from build123d import *

# Parameters (mm, degrees)
SKETCH1_W           = 153
SKETCH1_H           = 72
SKETCH1_R           = 2.5
BOSS_EXTRUDE1_DEPTH = 8
SKETCH2_R           = 4.5
SKETCH2_R_2         = 2.1
BOSS_EXTRUDE2_DEPTH = 5
CHAMFER1_SIZE       = 5
SKETCH3_R           = 2.1
CUT_EXTRUDE1_DEPTH  = 5


with BuildPart() as part:
    # Sketch1 → Boss-Extrude1 (new body)
    with BuildSketch(Plane.XY):
        with Locations((76.5, 36)):
            Rectangle(SKETCH1_W, SKETCH1_H)
        with Locations((21.5, 61)):
            Circle(SKETCH1_R, mode=Mode.SUBTRACT)
        with Locations(Location((21.5, 11, 0), (0, 0, 180))):
            Circle(SKETCH1_R, mode=Mode.SUBTRACT)
        with Locations(Location((131.5, 61, 0), (0, 0, 180))):
            Circle(SKETCH1_R, mode=Mode.SUBTRACT)
        with Locations((131.5, 11)):
            Circle(SKETCH1_R, mode=Mode.SUBTRACT)
        with Locations((61.5, 61)):
            Circle(SKETCH1_R, mode=Mode.SUBTRACT)
        with Locations((46.5, 61)):
            Circle(SKETCH1_R, mode=Mode.SUBTRACT)
        with Locations(Location((106.5, 61, 0), (0, 0, 180))):
            Circle(SKETCH1_R, mode=Mode.SUBTRACT)
        with Locations(Location((91.5, 61, 0), (0, 0, 180))):
            Circle(SKETCH1_R, mode=Mode.SUBTRACT)
    extrude(amount=BOSS_EXTRUDE1_DEPTH)

    # Sketch2 → Boss-Extrude2 (add)
    # profile 1 of 4: a face of its own
    with BuildSketch(Plane.XY.offset(8)):
        with Locations(Location((12.5, 59.5, 0), (0, 0, 180))):
            Circle(SKETCH2_R)
        with Locations((12.5, 59.5)):
            Circle(SKETCH2_R_2, mode=Mode.SUBTRACT)
    # profile 2 of 4: a face of its own
    with BuildSketch(Plane.XY.offset(8)):
        with Locations(Location((12.5, 12.5, 0), (0, 0, 180))):
            Circle(SKETCH2_R)
        with Locations(Location((12.5, 12.5, 0), (0, 0, 180))):
            Circle(SKETCH2_R_2, mode=Mode.SUBTRACT)
    # profile 3 of 4: a face of its own
    with BuildSketch(Plane.XY.offset(8)):
        with Locations(Location((140.5, 59.5, 0), (0, 0, 180))):
            Circle(SKETCH2_R)
        with Locations(Location((140.5, 59.5, 0), (0, 0, 180))):
            Circle(SKETCH2_R_2, mode=Mode.SUBTRACT)
    # profile 4 of 4: a face of its own
    with BuildSketch(Plane.XY.offset(8)):
        with Locations(Location((140.5, 12.5, 0), (0, 0, 180))):
            Circle(SKETCH2_R)
        with Locations((140.5, 12.5)):
            Circle(SKETCH2_R_2, mode=Mode.SUBTRACT)
    extrude(amount=BOSS_EXTRUDE2_DEPTH)

    # Chamfer1
    chamfer1_edges = [part.edges().sort_by_distance(p)[0] for p in [
        (0, 72, 4),
        (153, 72, 4),
        (153, 0, 4),
        (0, 0, 4),
    ]]
    chamfer(chamfer1_edges, length=CHAMFER1_SIZE)

    # Sketch3 → Cut-Extrude1 (cut)
    with BuildSketch(Plane.XY.offset(8)):
        with Locations((5.5, 6)):
            Circle(SKETCH3_R)
        with Locations(Location((5.5, 66, 0), (0, 0, 180))):
            Circle(SKETCH3_R)
        with Locations(Location((147.5, 6, 0), (0, 0, 180))):
            Circle(SKETCH3_R)
        with Locations((147.5, 66)):
            Circle(SKETCH3_R)
    extrude(amount=-CUT_EXTRUDE1_DEPTH, mode=Mode.SUBTRACT)


solid = part.part
Could you check a few things on this model? Use its own coordinates, in mm. A direction names the side the tool comes from. Give positions to 0.01 mm unless a question says otherwise; leave off trailing zeros. Order: outer loops, then holes, each group sorted by start corner. A loop starts at its lowest first (then second) coordinate and runs counter-clockwise, first axis right, second up.
Item 1: If we section it at C-C, the plane y = 40: Write out the boundary of the cut face in (x, z), plus the area to 3 significant figures.
Item 2: If we section it at B-B, the plane x = 91.5: Write out the boundary of the cut face in (y, z), plus the area to 3 significant figures.
Item 3: For faces 1 (the face through (129.115, 60.249, 3.944)), 2 (the face through (12, 13, 8)), which set-ups out of +Z, -Z, +X, -X, +Y, -Y let a thin tool reach every point of the face, with its end or its side?
Item 4: If we section it at D-D, the plane x = 117.5: Write out the boundary of the cut face in (y, z).
Item 5: I need wall thicknesses on line 1 (Y direction, x = 21.5, z = 1.75); line 2 (Y direction, x = 5.5, z = 6.15); line 3 (Z direction, x = 139, y = 53.5). Which ranges of each line are inside material? Lowest first, please.
Item 6: If we mould it in two halves opening along Y, with no side actions, what happens to faces 3 (the face through (143, 13, 13)), 4 (the face through (147, 66, 3)), 5 (the face through (151, 3, 4))? For each: pulls with the +Y half, pulls with the -Y half, needs draft (parallel to the pull), parting line crosses it, or undercut.
Item 7: I'm going to push flat-ended pins straight in: pin 1 (1 mm diameter, centred on x = 71, y = 58, fed in from +Z); pin 2 (6.5 mm diameter, centred on x = 140.5, y = 59.5, fed in from -Z); pin 3 (3 mm diameter, centred on x = 61.5, y = 61, fed in from +Z); pin 4 (4 mm diameter, centred on x = 5.5, y = 6, fed in from +Z). Where does each tip first touch, or does it pass through?
Item 8: If we section it at A-A, the plane z = 10.75: Write out the boundary of the cut face in (x, y).
Values:
1. outline: (0, 0) - (153, 0) - (153, 8) - (0, 8) - close
1. area: 1,220 mm2
2. outline: (0, 0) - (58.5, 0) - (58.5, 8) - (0, 8) - close; (63.5, 0) - (72, 0) - (72, 8) - (63.5, 8) - close
2. area: 536 mm2
3. face 1: +Z, -Z
3. face 2: +Z
4. outline: (0, 0) - (72, 0) - (72, 8) - (0, 8) - close
5. line 1: y = 0 to 8.5, 13.5 to 58.5, 63.5 to 72
5. line 2: y = 0 to 3.9, 8.1 to 63.9, 68.1 to 72
5. line 3: z = 0 to 8
6. face 3: needs draft
6. face 4: undercut
6. face 5: pulls with the -Y half
7. pin 1: stops at z = 8
7. pin 2: stops at z = 0
7. pin 3: passes through
7. pin 4: stops at z = 3
8. outline: circle Ø9 at (12.5, 12.5); circle Ø9 at (12.5, 59.5); circle Ø9 at (140.5, 12.5); circle Ø9 at (140.5, 59.5); hole circle Ø4.2 at (12.5, 12.5); hole circle Ø4.2 at (12.5, 59.5); hole circle Ø4.2 at (140.5, 12.5); hole circle Ø4.2 at (140.5, 59.5)
